from build123d import *

# Parameters (mm, degrees)
SKETCH2_W               = 109.5
SKETCH2_H               = 12.5
BOSS_EXTRUDE1_DEPTH     = 15
BOSS_EXTRUDE2_DEPTH     = 9.5
BOSS_EXTRUDE3_DEPTH     = 13
CUT_EXTRUDE2_DEPTH      = 149.758193052
CUT_EXTRUDE2_DEPTH_BACK = 149.758193052
FILLET2_R               = 2.5


with BuildPart() as part:
    # Sketch2 → Boss-Extrude1 (new, symmetric)
    with BuildSketch(Plane.XY):
        with Locations((54.75, 6.25)):
            Rectangle(SKETCH2_W, SKETCH2_H)
    extrude(amount=BOSS_EXTRUDE1_DEPTH, both=True)

    # Sketch2<3> → Boss-Extrude2 (add, symmetric)
    with BuildSketch(Plane.XY):
        Polygon((0, 48), (0, 12.5), (109.5, 12.5), (114.5, 12.5), (133, 31), (105, 31), (105, 48), align=None)
        with BuildLine():
            ThreePointArc((30.5, 25), (25, 30.5), (30.5, 36))
            Line((30.5, 36), (81.5, 36))
            ThreePointArc((81.5, 36), (87, 30.5), (81.5, 25))
            Line((81.5, 25), (30.5, 25))
        make_face(mode=Mode.SUBTRACT)
    extrude(amount=BOSS_EXTRUDE2_DEPTH, both=True)

    # Sketch2<4> → Boss-Extrude3 (add, symmetric)
    with BuildSketch(Plane.XY):
        Polygon((140, 48), (105, 48), (105, 31), (133, 31), (140, 38), align=None)
    extrude(amount=BOSS_EXTRUDE3_DEPTH, both=True)

    # Sketch3 → Cut-Extrude2 (cut, two sides: drawn at the far end of the back side and taken through both)
    with BuildSketch(Plane(origin=(0, 48, 0), x_dir=(1, 0, 0), z_dir=(0, 1, 0)).offset(-CUT_EXTRUDE2_DEPTH_BACK)):
        Polygon((-292.434063101, -3.5), (0, -3.5), (6.5, -3.5), (6.5, -15), (6.5, -307.434063101), (-410.479849846, -717.554203878), (-709.413912948, -413.620140776), align=None)
    extrude(amount=CUT_EXTRUDE2_DEPTH + CUT_EXTRUDE2_DEPTH_BACK, mode=Mode.SUBTRACT)

    # Fillet2
    fillet2_edges = [part.edges().sort_by_distance(p)[0] for p in [
        (87, 30.5, 9.5),
        (56, 25, 9.5),
        (25, 30.5, 9.5),
        (56, 36, 9.5),
    ]]
    fillet(fillet2_edges, radius=FILLET2_R)

    # Mirror3: part across plane


with BuildPart() as part_1:
    add(part.part)
    add(part.part.mirror(Plane(origin=(0, 0, 15), x_dir=(0, 0, 1), z_dir=(0, -1, 0))))


solid = part_1.part
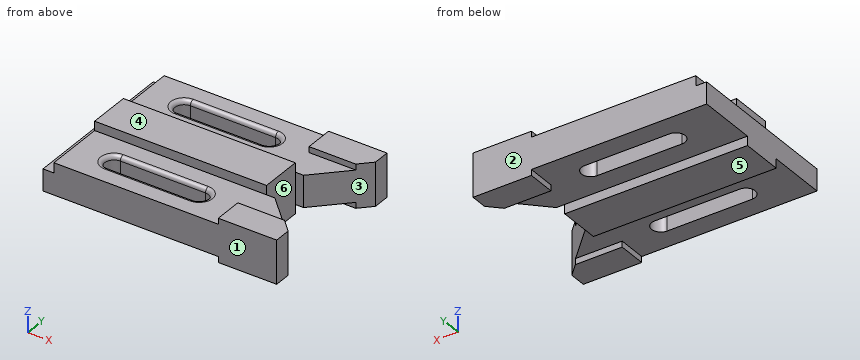
Work out the finished part from the listing and answer in its coordinate system (mm). Face numbers are marked on the shaded views. A direction names the side the tool comes from. Round coordinates to 2 decimals unless told otherwise and drop trailing zeros. Write each loop counter-clockwise with the first axis right and the second up, starting at its lowest first coordinate (ties: lowest second). Pieces come first, ordered by that corner, then holes.
1) A cutting plane is placed at B-B (z = -2). Give the vertices of the cut face in (x, y).
2) The mould has two halves that part along Y. Classify the marked faces 1, 2, 3 and 4: pulls with the +Y half, pulls with the -Y half, needs draft (parallel to the pull), parting line crosses it, or undercut.
3) Straight lines are drawn through the part: line 1 (Y direction, x = 66, z = -7.5); line 2 (Y direction, x = 112, z = -9.75); line 3 (Y direction, x = 67, z = 10.25). For each, find the intervals that lie inside material, in ascending order.
4) A cutting plane is placed at C-C (x = 98). Give the vertices of the cut face in (y, z).
5) Given pin 1 Ø1 at (x, z) = (48, 11) entering from -Y; pin 2 Ø8 at (x, y) = (86.5, 18) entering from +Z; pin 3 Ø3 at (y, z) = (-43, 10.5) entering from -X; pin 4 Ø10 at (y, z) = (20, 2.5) entering from -X, each flat-ended and moving along its own axis, determine where each tip first touches the part or whether it passes through.
6) A tool of negligible diameter and unlimited length cuts with its end or side. For the marked faces 5 and 6, from which of +Z, -Z, +X, -X, +Y, -Y can it reach the whole face along a straight path? Write none if from no direction.
7) A cutting plane is placed at A-A (x = 33.5). Give the vertices of the cut face in (y, z), plus the area to 3 significant figures.
Completed:
1. outline: (0, -48) - (140, -48) - (140, -38) - (114.5, -12.5) - (109.5, -12.5) - (109.5, 12.5) - (114.5, 12.5) - (140, 38) - (140, 48) - (0, 48) - close; hole (30.5, -36) - (81.5, -36) arc R5.5 ccw to (81.5, -25) - (30.5, -25) arc R5.5 ccw to start; hole (30.5, 25) - (81.5, 25) arc R5.5 ccw to (81.5, 36) - (30.5, 36) arc R5.5 ccw to start
2. face 1: pulls with the -Y half
2. face 2: pulls with the +Y half
2. face 3: undercut
2. face 4: needs draft
3. line 1: y = -48 to -36, -25 to 25, 36 to 48
3. line 2: y = -48 to -31, 31 to 48
3. line 3: y = -12.5 to 12.5
4. outline: (-48, -9.5) - (-12.5, -9.5) - (-12.5, -15) - (12.5, -15) - (12.5, -9.5) - (48, -9.5) - (48, 9.5) - (12.5, 9.5) - (12.5, 15) - (-12.5, 15) - (-12.5, 9.5) - (-48, 9.5) - close
5. pin 1: stops at y = -12.5
5. pin 2: stops at z = 9.5
5. pin 3: stops at x = 6.5
5. pin 4: stops at x = 0
6. face 5: -Z, +X, -X, +Y, -Y
6. face 6: +Z, -Z, +X
7. outline: (-48, -9.5) - (-36, -9.5) - (-36, 7) arc R2.5 ccw to (-38.5, 9.5) - (-48, 9.5) - close; (-25, -9.5) - (-12.5, -9.5) - (-12.5, -15) - (12.5, -15) - (12.5, -9.5) - (25, -9.5) - (25, 7) arc R2.5 ccw to (22.5, 9.5) - (12.5, 9.5) - (12.5, 15) - (-12.5, 15) - (-12.5, 9.5) - (-22.5, 9.5) arc R2.5 ccw to (-25, 7) - close; (36, -9.5) - (48, -9.5) - (48, 9.5) - (38.5, 9.5) arc R2.5 ccw to (36, 7) - close
7. area: 1,680 mm2
